Geometry check sheet. Reference: drawing and pictorial views, mm from the part's lowest x, y, z. A direction names the side the tool comes from. Round coordinates to 2 decimals unless told otherwise and drop trailing zeros. Order: outer loops, then holes, each group sorted by start corner. A loop starts at its lowest first (then second) coordinate and runs counter-clockwise, first axis right, second up.
(1) Sectioned sample at B-B (y = 5.75). Give the number of separate pieces and of enclosed holes in the cut face, plus the area to 3 significant figures.
(2) Sectioned sample at A-A (x = 2.3). Record the boundary of the cut face in (y, z) (3 decimals).
(3) Sectioned sample at D-D (x = 15.5). Record the boundary of the cut face in (y, z), plus the area to 3 significant figures.
(4) Sectioned sample at C-C (z = 16.75). Record the boundary of the cut face in (x, y) (3 decimals), plus the area to 3 significant figures.
(5) Go/stop test with flat-tipped pins: pin 1 (1.4 mm diameter, centred on x = 29.5, y = 4.5, fed in from +Z); pin 2 (4 mm diameter, centred on y = 9, z = 19.5, fed in from -X); pin 3 (1.1 mm diameter, centred on y = 8, z = 21, fed in from +X); pin 4 (2.5 mm diameter, centred on x = 30.5, y = 4.5, fed in from -Z). Record where each tip stops, or that it passes through.
(6) Set-up check for the marked faces 1, 2, 3 and 4: record each of +Z, -Z, +X, -X, +Y, -Y from which the full face is reachable in a straight line by a thin tool's end or side.
(7) Material ranges on line 1 along Y through (x, z) = (2.3, 17.6) (3 decimals); line 2 along X through (y, z) = (3.5, 11.5); line 3 along Z through (x, y) = (8.5, 3.75), recorded low to high.
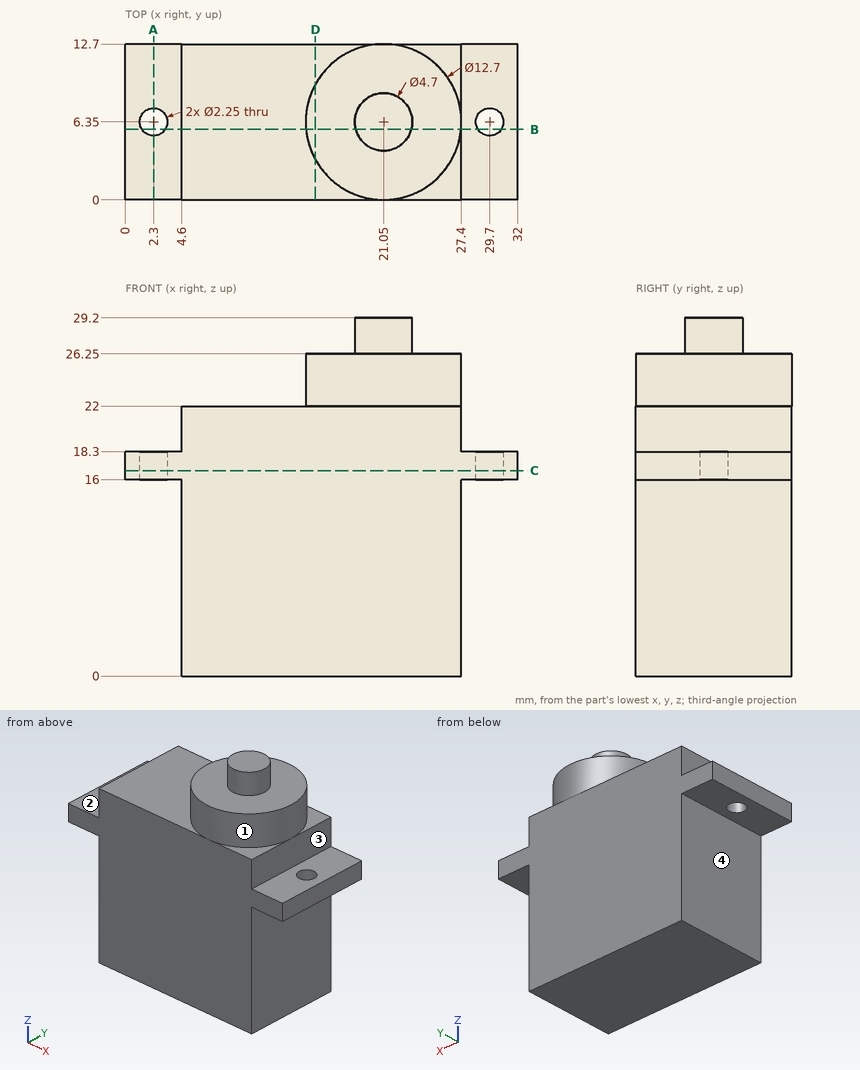
Answer below:
1. separate pieces: 3
1. enclosed holes: 0
1. area: 581 mm2
2. outline: (0, 16) - (5.225, 16) - (5.225, 18.3) - (0, 18.3) - close; (7.475, 16) - (12.7, 16) - (12.7, 18.3) - (7.475, 18.3) - close
3. outline: (0, 0) - (12.7, 0) - (12.7, 22) - (9.44, 22) - (9.44, 26.25) - (3.26, 26.25) - (3.26, 22) - (0, 22) - close
3. area: 306 mm2
4. outline: (0, 0) - (32, 0) - (32, 12.7) - (0, 12.7) - close; hole circle Ø2.25 at (2.3, 6.35); hole circle Ø2.25 at (29.7, 6.35)
4. area: 398 mm2
5. pin 1: stops at z = 18.3
5. pin 2: stops at x = 0
5. pin 3: stops at x = 27.4
5. pin 4: stops at z = 16
6. face 1: +Z
6. face 2: +Z, -X, +Y, -Y
6. face 3: +Z, +X, +Y, -Y
6. face 4: -Z, -X, +Y, -Y
7. line 1: y = 0 to 5.225, 7.475 to 12.7
7. line 2: x = 4.6 to 27.4
7. line 3: z = 0 to 22
